Answer from the drawing. Dimensions are ordinates in mm from the lowest x, y and z of the part. A direction names the side the tool comes from. Round coordinates to 2 decimals unless told otherwise and drop trailing zeros. Loops run counter-clockwise (first coordinate to the right, second up) from the corner with the lowest first, then second, coordinate; pieces in that order, holes last. Notation, with made-up numbers: (54.25, 16.5) - (76.25, 16.5) arc R19 ccw to (76.25, 26.5) - close; hole circle Ø1 at (85.5, -15.75). An arc over 180 degrees is marked (long way). Answer as CSV lines item,"result". Start each with the question number.
Q1. Section D-D on x = 8.75 is taken. Write down the section's boundary in (y, z), then the cut area to 3 significant figures.
Q2. For the marked faces 1 and 2, determine the directions among +Z, -Z, +X, -X, +Y, -Y from which every point of the face is accessible in a straight line to the end or side of a thin tool.
Q3. Section C-C on z = 13.25 is taken. Write down the section's boundary in (x, y).
Q4. Section B-B on y = 29 is taken. Write down the section's boundary in (x, z), then the cut area to 3 significant figures.
Q5. Each of these flat-tipped pins is pushed along its axis until it touches: pin 1 Ø12.5 at (x, y) = (6.5, 19.5) entering from -Z; pin 2 Ø4 at (x, y) = (16.5, 4.5) entering from -Z; pin 3 Ø1 at (x, z) = (19, 6) entering from +Y. Where does it stop, or does it pass through?
Q6. Section A-A on x = 2 is taken. Write down the section's boundary in (y, z), then the cut area to 4 significant figures.
Q7. Straight lines are drawn through the part: L1, parallel to Y at x = 19.25, z = 14; L2, parallel to Z at x = 17.75, y = 30; L3, parallel to Y at x = 9.25, z = 16. For each, find the intervals that lie inside material, in ascending order. Write a range as [from, to].
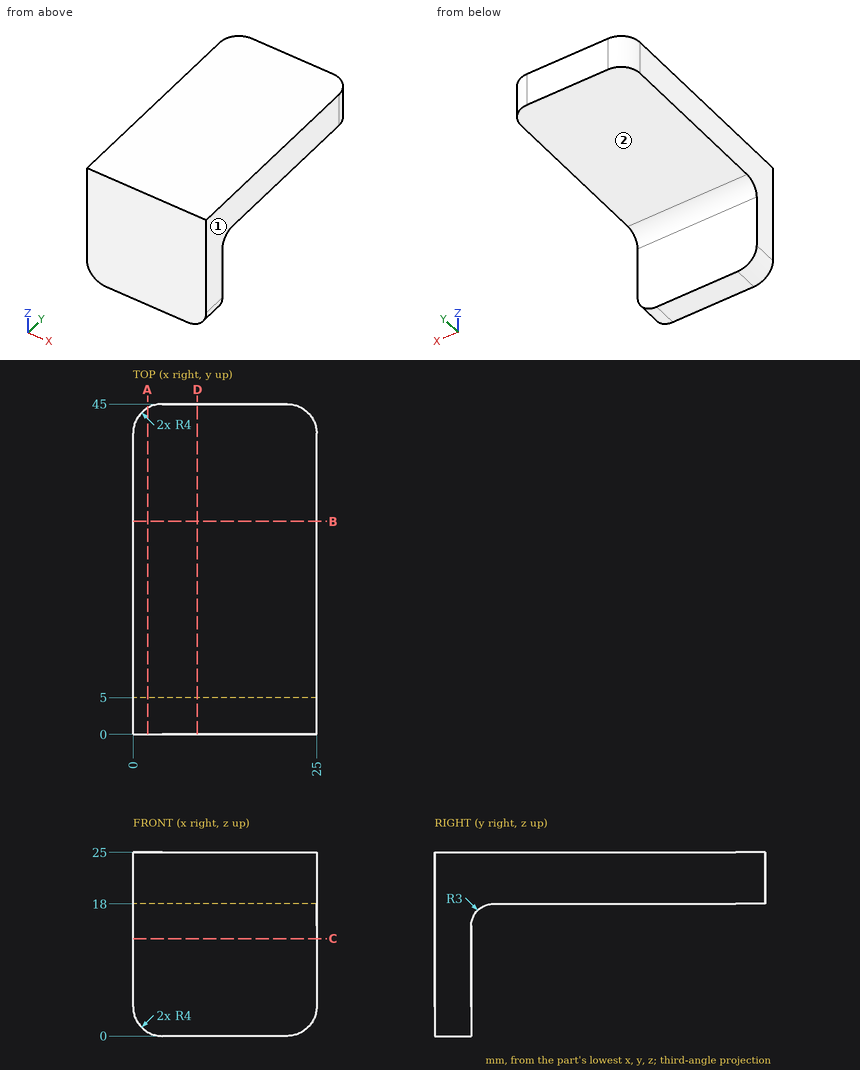
Findings:
1,outline,"(0, 0) - (5, 0) - (5, 15) arc R3 cw to (8, 18) - (45, 18) - (45, 25) - (0, 25) - close"
1,area,"407 mm^2"
2,face 1,"+Z, -Z, +X, +Y, -Y"
2,face 2,"-Z, +X, -X, +Y"
3,outline,"(0, 0) - (25, 0) - (25, 5) - (0, 5) - close"
4,outline,"(0, 18) - (25, 18) - (25, 25) - (0, 25) - close"
4,area,"175 mm^2"
5,pin 1,"stops at z = 18"
5,pin 2,"stops at z = 0"
5,pin 3,"stops at y = 5"
6,outline,"(0, 0.54) - (5, 0.54) - (5, 15) arc R3 cw to (8, 18) - (44.46, 18) - (44.46, 25) - (0, 25) - close"
6,area,"400.5 mm^2"
7,L1,"y = [0, 5]"
7,L2,"z = [18, 25]"
7,L3,"y = [0, 5.17]"
